For this review, take the finished solid that the model builds, in its own axes (mm). A direction names the side the tool comes from. Coordinates: 2 decimals unless noted, no trailing zeros. Loops run counter-clockwise (first coordinate to the right, second up) from the corner with the lowest first, then second, coordinate; pieces in that order, holes last.
1. Clearance check with flat-ended pins moving along their axes: P1, Ø4, axis at y = -4.5, z = 12, coming from the +X side; P2, Ø4, axis at y = -3, z = 16.5, coming from the +X side; P3, Ø6, axis at x = -8.5, z = 17, coming from the -Y side. State where each tip first meets the part, or that it passes through.
2. Machinability: for faces 1 (the face through (-0.16, -4.63, 10.76)), 2 (the face through (-15.075, 4, 17)), which of the approach directions +Z, -Z, +X, -X, +Y, -Y give a long, thin tool a straight path to every point of the face, cutting with its end or side? Answer none if there is none.
3. Take a section at B-B, the plane x = 10. State the section outline as (y, z) points (3 decimals).
4. Take a section at A-A, the plane z = 17. State the section outline as (x, y) points (3 decimals), then the cut area to 3 significant figures.
5. To check wall thickness, follow probe 1 along Y at (x, z) = (13.5, 11.5); probe 2 along Z at (x, y) = (1, -3.75); probe 3 along Z at (x, y) = (0.5, 1.75). State the ranges of each line that lie inside material, in increasing order.
6. Take a section at C-C, the plane x = 6. State the section outline as (y, z) points (3 decimals).
7. Mouldability with a two-part tool opening along Y and no side actions: class faces 3 (the face through (0.672, -16.554, 16.965)), 4 (the face through (0, 4, 24.575)), 5 (the face through (0, 5, 17)) as pulls with the +Y half, pulls with the -Y half, needs draft (parallel to the pull), parting line crosses it, or undercut.
```python
from build123d import *

# Parameters (mm, degrees)
PAD003_DEPTH        = 1.5
HOLE001_D           = 3
HOLE001_DEPTH       = 25
HOLE001_CSINK_D     = 6.1
HOLE001_CSINK_ANGLE = 90
SKETCH009_R         = 1.25


with BuildPart() as part:
    # Sketch006 → Pad003 (new body)
    with BuildSketch(Plane.XZ):
        with BuildLine():
            Line((-15.075, 6.075), (-15.075, -6.075))
            ThreePointArc((-15.075, -6.075), (-14.63566, -7.13566), (-13.575, -7.575))
            Line((-13.575, -7.575), (13.575, -7.575))
            ThreePointArc((13.575, -7.575), (14.63566, -7.13566), (15.075, -6.075))
            Line((15.075, -6.075), (15.075, 6.075))
            ThreePointArc((15.075, 6.075), (14.63566, 7.13566), (13.575, 7.575))
            Line((13.575, 7.575), (-13.575, 7.575))
            ThreePointArc((-13.575, 7.575), (-14.63566, 7.13566), (-15.075, 6.075))
        make_face()
    extrude(amount=PAD003_DEPTH)

    # Hole001
    with Locations(Plane.XZ.offset(1.5)):
        with Locations((-10, 0), (10, 0)):
            CounterSinkHole(HOLE001_D / 2, HOLE001_CSINK_D / 2, depth=HOLE001_DEPTH, counter_sink_angle=HOLE001_CSINK_ANGLE)

    # AdditivePipe: sweep along a path in Sketch008
    with BuildLine(Plane.YZ) as additivepipe_path:
        Line((-1.5, 5), (-18, 5))
        ThreePointArc((-18, 5), (-19.767767, 4.267767), (-20.5, 2.5))
        Line((-20.5, 2.5), (-20.5, -2.5))
        ThreePointArc((-20.5, -2.5), (-19.767767, -4.267767), (-18, -5))
        Line((-18, -5), (-1.5, -5))
    # Sketch009 (on Face5 of Hole001) → AdditivePipe (sweep)
    with BuildSketch(Plane.XZ.offset(1.5)):
        with Locations((0, -5)):
            Circle(SKETCH009_R)
    sweep(path=additivepipe_path.line)


with BuildPart() as part_1:
    # Body001 placement: moved
    add(part.part.moved(Location((0, 5, 17))))


solid = part_1.part
```
Results list:
1. P1: stops at x = 1.25
1. P2: passes through
1. P3: stops at y = 3.5
2. face 1: none
2. face 2: +Z, -Z, -X, +Y, -Y
3. outline: (3.5, 9.425) - (5, 9.425) - (5, 15.45) - (3.5, 13.95) - close; (3.5, 20.05) - (5, 18.55) - (5, 24.575) - (3.5, 24.575) - close
4. outline: (-15.075, 3.5) - (-13.05, 3.5) - (-11.55, 5) - (-15.075, 5) - close; (-8.45, 5) - (-6.95, 3.5) - (6.95, 3.5) - (8.45, 5) - close; circle Ø2.5 at (0, -15.5); (11.55, 5) - (13.05, 3.5) - (15.075, 3.5) - (15.075, 5) - close
4. area: 36.3 mm2
5. probe 1: y = 3.5 to 5
5. probe 2: z = 11.25 to 12.75, 21.25 to 22.75
5. probe 3: z = 10.85 to 13.15, 20.85 to 23.15
6. outline: (3.5, 9.425) - (5, 9.425) - (5, 24.575) - (3.5, 24.575) - close
7. face 3: undercut
7. face 4: needs draft
7. face 5: pulls with the +Y half
